Could you check a few things on this drawing? It's one solid part, dimensions in mm from its lowest x, y, z. Give positions to 0.01 mm unless a question says otherwise; leave off trailing zeros. Loops run counter-clockwise (first coordinate to the right, second up) from the corner with the lowest first, then second, coordinate; pieces in that order, holes last.
1. I need wall thicknesses on line 1 along Y through (x, z) = (85, 1.35); line 2 along X through (y, z) = (185, 3.45); line 3 along Y through (x, z) = (57, 0.7). Which ranges of each line are inside material? Lowest first, please.
2. Imagine slicing it at A-A (x = 115). List the corners of the cut face in (y, z) for me.
3. Imagine slicing it at B-B (y = 65). List the corners of the cut face in (x, z) for me.
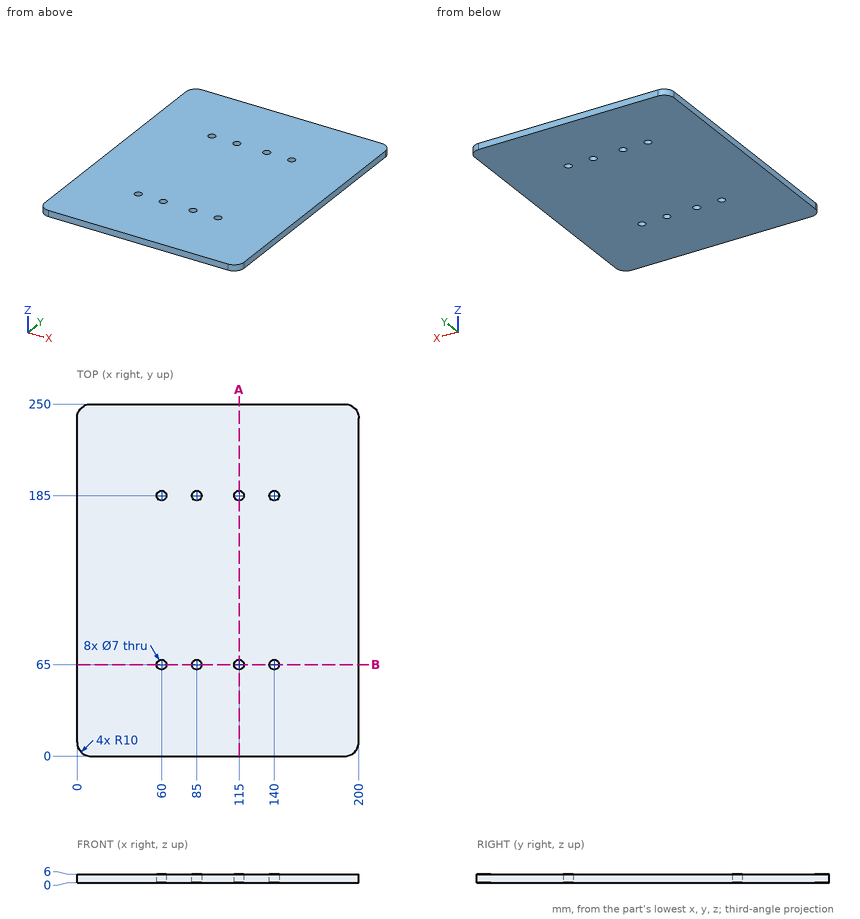
Derived:
1. line 1: y = 0 to 61.5, 68.5 to 181.5, 188.5 to 250
1. line 2: x = 0 to 56.5, 63.5 to 81.5, 88.5 to 111.5, 118.5 to 136.5, 143.5 to 200
1. line 3: y = 0 to 63.2, 66.8 to 183.2, 186.8 to 250
2. outline: (0, 0) - (61.5, 0) - (61.5, 6) - (0, 6) - close; (68.5, 0) - (181.5, 0) - (181.5, 6) - (68.5, 6) - close; (188.5, 0) - (250, 0) - (250, 6) - (188.5, 6) - close
3. outline: (0, 0) - (56.5, 0) - (56.5, 6) - (0, 6) - close; (63.5, 0) - (81.5, 0) - (81.5, 6) - (63.5, 6) - close; (88.5, 0) - (111.5, 0) - (111.5, 6) - (88.5, 6) - close; (118.5, 0) - (136.5, 0) - (136.5, 6) - (118.5, 6) - close; (143.5, 0) - (200, 0) - (200, 6) - (143.5, 6) - close
